Autodesk Inventor part; units mm, degrees
ref_plane "YZ Plane" through (0, 0, 0) normal (1, 0, 0) x (0, 1, 0)
ref_plane "XZ Plane" through (0, 0, 0) normal (0, 1, 0) x (-1, 0, 0)
ref_plane "XY Plane" through (0, 0, 0) normal (0, 0, 1) x (1, 0, 0)
sketch "Sketch1" plane through (0, 0, 0) normal (0, 0, 1) x (1, 0, 0)
  circle A0 centre (0, 0) radius 3.175
  dimension "d0" = 6.35
extrude "Extrusion1" add sketch "Sketch1" along normal blind 57.15
sketch "Sketch2" plane through (0, 0, 0) normal (0, 0, -1) x (-1, 0, 0)
  circle A0 centre (0, 0) radius 3.175
  circle A1 centre (0, 0) radius 4.7625
  dimension "d3" = 9.525
extrude "Extrusion2" add sketch "Sketch2" along normal blind 6.35 contours A0 | A1
sketch "Sketch3" plane through (0, 0, -6.35) normal (0, 0, -1) x (-1, 0, 0)
  circle A0 centre (0, 0) radius 4.7625
  line L0 (-1.3748, 2.3812) -> (1.3748, 2.3813)
  line L1 (1.3748, 2.3813) -> (2.7496, 0)
  line L2 (2.7496, 0) -> (1.3748, -2.3812)
  line L3 (1.3748, -2.3812) -> (-1.3748, -2.3812)
  line L4 (-1.3748, -2.3812) -> (-2.7496, 0)
  line L5 (-2.7496, 0) -> (-1.3748, 2.3812)
  dimension "d6" = 4.7625
extrude "Extrusion3" cut sketch "Sketch3" against normal blind 3.175 contours L0 L1 L2 L3 L4 L5
chamfer "Chamfer1" distance 0.508 angle 45 3 edges at (-3.175, 0, 57.15) (4.7625, 0, 0) (4.7625, 0, -6.35)
thread "Thread1"
properties part number "14-20 x2500" material "Steel"
The listing builds one solid part. Answer for the finished solid, in the listing's coordinates (mm). A direction names the side the tool comes from. Round coordinates to 2 decimals unless told otherwise and drop trailing zeros. Write each loop counter-clockwise with the first axis right and the second up, starting at its lowest first coordinate (ties: lowest second). Pieces come first, ordered by that corner, then holes. Notation, with made-up numbers: (76, -17.5) - (116, -17.5) arc R14 ccw to (116, -1.5) - close; hole circle Ø5 at (79.25, -36). An arc over 180 degrees is marked (long way). Use one line per item in the form item = value. Start each with the question number.
Item 1: Find the intervals of material crossed by line 1 (Z direction, x = 0, y = -1.25) (3 decimals); line 2 (Z direction, x = 2.75, y = -2.25); line 3 (Y direction, x = 0.25, z = 3.5), in increasing order. Write a range as [from, to].
Item 2: Determine the mould class of faces 4 (the cylindrical face through (3.78, 2.9, -3.14)), 5 (the flat face through (2, -3, 0)), 6 (the flat face through (2.05, -1.21, -4.78)) for opening direction Y: +Y half, -Y half, draft (parallel to the pull), parting line (faces both ways), or undercut.
Item 3: A cutting plane is placed at A-A (z = 36). Write down the section's boundary in (x, y) (3 decimals).
Item 4: A tool of negligible diameter and unlimited length cuts with its end or side. For faces 1 (the flat face through (0, 0, -3.175)), 2 (the cylindrical face through (-0.69, 3.1, 27.92)), 3 (the flat face through (-2, -2, -6.35)), from which of +Z, -Z, +X, -X, +Y, -Y can it reach the whole face along a straight path? Write none if from no direction.
Item 5: Flat-ended cylindrical pins translate along their axes: pin 1 Ø5 at (y, z) = (2.5, 3) entering from -X (3 decimals); pin 2 Ø3 at (x, z) = (-0.5, 30) entering from +Y (3 decimals); pin 3 Ø1.5 at (y, z) = (2, 48.5) entering from -X. Find the tip coordinate at first contact, or state that the pin passes through.
The answers:
q1.line_1 = [-3.175, 57.15]
q1.line_2 = [-6.35, 0]
q1.line_3 = [-3.17, 3.17]
q2.face_4 = parting line
q2.face_5 = draft
q2.face_6 = undercut
q3.outline = circle Ø6.35 at (0, 0)
q4.face_1 = -Z
q4.face_2 = +Z
q4.face_3 = -Z, +X, -X, +Y, -Y
q5.pin_1 = -3.175
q5.pin_2 = 3.175
q5.pin_3 = -2.92
